```python
from build123d import *

# Parameters (mm, degrees)
SKETCH1_W                    = 48
SKETCH1_H                    = 0.5
BASE_FLANGE1_DEPTH           = 211
SKETCH6_R                    = 1.75
CUT_EXTRUDE1_DEPTH           = 10
EDGE_FLANGE1_STRIP_CUT_DEPTH = 422
EDGE_FLANGE1_DEPTH           = 422
HEM1_START                   = -211
HEM1_DEPTH                   = 422
HEM1_2_DEPTH                 = 422


# Read off the part's stored shape, not the designer's step: Hem1
# Sheet-metal steps are written as plain solids
with BuildPart() as part:
    # Sketch1 → Base-Flange1 (new, symmetric)
    with BuildSketch(Plane.XY):
        with Locations((24, -0.25)):
            Rectangle(SKETCH1_W, SKETCH1_H)
    extrude(amount=BASE_FLANGE1_DEPTH, both=True)

    # Sketch6 → Cut-Extrude1 (cut)
    with BuildSketch(Plane(origin=(0, 0, 0), x_dir=(1, 0, 0), z_dir=(0, 1, 0))):
        with Locations(Location((5, 196, 0), (0, 0, 270))):
            Circle(SKETCH6_R)
        with Locations(Location((5, 0, 0), (0, 0, 270))):
            Circle(SKETCH6_R)
        with Locations(Location((5, -196, 0), (0, 0, 270))):
            Circle(SKETCH6_R)
    extrude(amount=-CUT_EXTRUDE1_DEPTH, mode=Mode.SUBTRACT)

    # Edge-Flange1 strip (across the edge) → Edge-Flange1 strip cut (cut)
    with BuildSketch(Plane(origin=(48, -0.5, -211), x_dir=(-0.6560590289905086, 0.754709580222771, 0), z_dir=(0, 0, 1))):
        Polygon((-4.886773951, -6.383716909), (2.13206437, 1.69053295), (1.75470958, 2.018562465), (-5.264128741, -6.055687395), align=None)
    extrude(amount=EDGE_FLANGE1_STRIP_CUT_DEPTH, mode=Mode.SUBTRACT)

    # Edge-Flange1 section (across the edge) → Edge-Flange1 (add)
    with BuildSketch(Plane(origin=(48, -0.5, -211), x_dir=(-0.6560590289905086, 0.754709580222771, 0), z_dir=(0, 0, 1))):
        with BuildLine():
            Line((-0.5, 2.674621494), (-0.5, 18))
            Line((-0.5, 18), (0, 18))
            Line((0, 18), (0, 2.674621494))
            ThreePointArc((0, 2.674621494), (0.649792619, 1.737949305), (1.75470958, 2.018562465))
            Line((1.75470958, 2.018562465), (2.13206437, 1.69053295))
            ThreePointArc((2.13206437, 1.69053295), (0.474688928, 1.26961321), (-0.5, 2.674621494))
        make_face()
    extrude(amount=EDGE_FLANGE1_DEPTH)

    # Hem1 outline → Hem1 (cut)
    with BuildSketch(Plane.XY.offset(HEM1_START)):
        with BuildLine():
            ThreePointArc((35.309289256, -12.19437304), (34.892198615, -12.374586092), (34.447599479, -12.280922038))
            Line((34.447599479, -12.280922038), (34.415227556, -12.309062522))
            Line((34.415227556, -12.309062522), (34.74325707, -12.686417312))
            Line((34.74325707, -12.686417312), (35.309289256, -12.19437304))
        make_face()
    extrude(amount=HEM1_DEPTH, mode=Mode.SUBTRACT)

    # Hem1 2 outline → Hem1 2 (add)
    with BuildSketch(Plane.XY.offset(HEM1_START)):
        with BuildLine():
            Line((41.634293844, -5.371117442), (41.306264329, -4.993762652))
            Line((41.306264329, -4.993762652), (34.325200712, -11.06230867))
            ThreePointArc((34.325200712, -11.06230867), (34.070999747, -11.703294486), (34.447599479, -12.280922038))
            Line((34.447599479, -12.280922038), (34.981259741, -11.81701825))
            ThreePointArc((34.981259741, -11.81701825), (34.628567589, -11.792355612), (34.653230227, -11.43966346))
            Line((34.653230227, -11.43966346), (41.634293844, -5.371117442))
        make_face()
    extrude(amount=HEM1_2_DEPTH)


solid = part.part
```
Geometry check sheet. Reference: the model listing, model coordinates, mm. A direction names the side the tool comes from. Coordinates: 2 decimals unless noted, no trailing zeros. Order: outer loops, then holes, each group sorted by start corner. A loop starts at its lowest first (then second) coordinate and runs counter-clockwise, first axis right, second up.
Item 1: Tool access check on faces 5 (the flat face through (30.2, -0.2, -211)), 6 (the flat face through (22, -0.5, 3)), 7 (the flat face through (38.09, -8.45, -2.95)). Record the directions out of +Z, -Z, +X, -X, +Y, -Y that give a thin tool (end or side, any length) a straight path to the whole face; none if there is none.
Item 2: Section check A-A (z = 172). Enter the section's corners in (x, y), plus the area to 3 significant figures.
Item 3: Mould release check, pull along Y, two halves, no side actions. Record for faces 1 (the flat face through (37.86, -7.99, -2.95)), 2 (the flat face through (30.2, -0.2, 211)), 3 (the flat face through (40.886, -7.346, -2.954)), 4 (the flat face through (22, 0, 3)): released by +Y, released by -Y, zero draft, split by the parting line, or undercut.
Item 4: Scan lines: line 1 along X through (y, z) = (-0.4, 196); line 2 along Y through (x, z) = (38.5, 190.5); line 3 along Y through (x, z) = (37, 183.5). Record each from-to range of solid material in increasing order.
Item 5: Depth check by flat-ended pin: pin 1 (5 mm diameter, centred on x = 22.5, z = -80.5, fed in from -Y); pin 2 (2 mm diameter, centred on y = -4.5, z = -28.5, fed in from +X); pin 3 (5 mm diameter, centred on y = -10, z = -70, fed in from +X). Enter the tip coordinate at first touch or a pass-through.
Check sheet entries:
1. face 5: -Z, +X, -X, +Y, -Y
1. face 6: +Z, -Z, -X
1. face 7: +Z, -Z
2. outline: (0, -0.5) - (45.33, -0.5) arc R1 cw to (45.98, -2.25) - (34.98, -11.82) arc R0.25 cw to (34.65, -11.44) - (41.63, -5.37) - (41.31, -4.99) - (34.33, -11.06) arc R0.75 ccw to (35.31, -12.19) - (46.31, -2.63) arc R1.5 ccw to (45.33, 0) - (0, 0) - close
2. area: 36.9 mm2
3. face 1: undercut
3. face 2: zero draft
3. face 3: released by -Y
3. face 4: released by +Y
4. line 1: x = 0 to 3.25, 6.75 to 46.35
4. line 2: y = -9.42 to -8.76, -8.1 to -7.43, -0.5 to 0
4. line 3: y = -10.72 to -10.06, -9.4 to -8.74, -0.5 to 0
5. pin 1: stops at y = -0.5
5. pin 2: stops at x = 45.31
5. pin 3: stops at x = 40.71
